Read the model definition and answer for the solid it produces. Units are mm, in the model's axes. Give positions to 0.01 mm unless a question says otherwise; leave off trailing zeros. Write each loop counter-clockwise with the first axis right and the second up, starting at its lowest first coordinate (ties: lowest second). Pieces come first, ordered by that corner, then holes. Notation, with made-up numbers: (32, -18) - (91, -18) arc R30 cw to (91, 5) - close; hole circle Ø2 at (33.5, 50.25). An arc over 180 degrees is marked (long way). Answer as CSV lines item,"result".
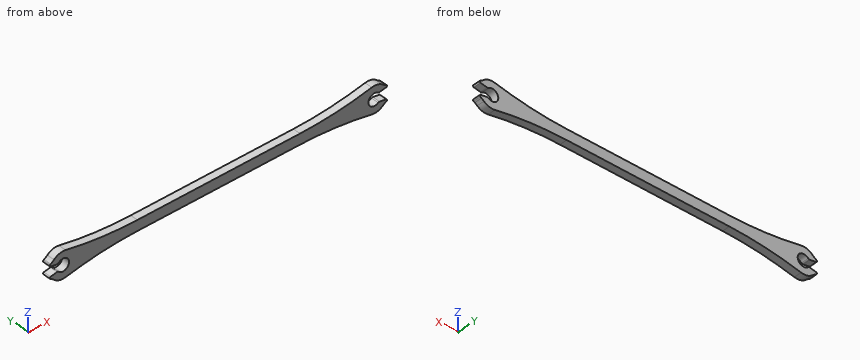
```python
from build123d import *

# Parameters (mm, degrees)
F1_DEPTH = 1.1
F2_R     = 0.3
F3_R     = 100
F4_R     = 0.5
F5_R     = 5


with BuildPart() as f1:
    # F0 (on Front) → F1 (new body, symmetric)
    with BuildSketch(Plane.XZ):
        with BuildLine():
            ThreePointArc((1.224745, -1.25), (-1.75, 0), (1.224745, 1.25))
            Line((1.224745, 1.25), (4.179168, 1.770945))
            Line((4.179168, 1.770945), (2.648788, 2.65451))
            ThreePointArc((2.648788, 2.65451), (-0.698939, 3.684289), (-3.436932, 1.5))
            Line((-3.436932, 1.5), (-86.563068, 1.5))
            ThreePointArc((-86.563068, 1.5), (-89.480722, 3.713873), (-92.893705, 2.385156))
            Line((-92.893705, 2.385156), (-94.390564, 1.520945))
            Line((-94.390564, 1.520945), (-91.436141, 1))
            ThreePointArc((-91.436141, 1), (-88.25, 0), (-91.436141, -1))
            Line((-91.436141, -1), (-94.390564, -1.520945))
            Line((-94.390564, -1.520945), (-92.893705, -2.385156))
            ThreePointArc((-92.893705, -2.385156), (-89.480722, -3.713873), (-86.563068, -1.5))
            Line((-86.563068, -1.5), (-3.436932, -1.5))
            ThreePointArc((-3.436932, -1.5), (-0.698939, -3.684289), (2.648788, -2.65451))
            Line((2.648788, -2.65451), (4.179168, -1.770945))
            Line((4.179168, -1.770945), (1.224745, -1.25))
        make_face()
    extrude(amount=F1_DEPTH, both=True)

    # F2
    f2_edges = [f1.edges().sort_by_distance(p)[0] for p in [
        (4.179168, 0, 1.770945),
        (4.179168, 0, -1.770945),
        (-94.390564, 0, -1.520945),
        (-94.390564, 0, 1.520945),
    ]]
    fillet(f2_edges, radius=F2_R)

    # F3
    f3_edges = [f1.edges().sort_by_distance(p)[0] for p in [
        (-3.436932, 0, 1.5),
        (-3.436932, 0, -1.5),
        (-86.563068, 0, 1.5),
        (-86.563068, 0, -1.5),
    ]]
    fillet(f3_edges, radius=F3_R)

    # F4
    f4_edges = [f1.edges().sort_by_distance(p)[0] for p in [
        (1.224745, 0, 1.25),
        (1.224745, 0, -1.25),
        (-91.436141, 0, 1),
        (-91.436141, 0, -1),
    ]]
    fillet(f4_edges, radius=F4_R)

    # F5
    f5_edges = [f1.edges().sort_by_distance(p)[0] for p in [
        (2.648788, 0, 2.65451),
        (2.648788, 0, -2.65451),
        (-92.893705, 0, -2.385156),
        (-92.893705, 0, 2.385156),
    ]]
    fillet(f5_edges, radius=F5_R)


solid = f1.part
```
(1) Each of these flat-tipped pins is pushed along its axis until it touches: P1, Ø2, axis at x = -90, z = 0, coming from the +Y side; P2, Ø1.1, axis at x = -45, y = 0, coming from the -Z side. Where does it stop, or does it pass through?
Worked out:
P1,"passes through"
P2,"stops at z = -1.5"
(2) Find the intervals of material crossed by L1, parallel to Z at x = 0, y = 0.1; L2, parallel to X at y = -0.4, z = 0; L3, parallel to Z at x = -45.5, y = 0.1, in increasing order.
Worked out:
L1,"z = -3.75 to -1.75, 1.75 to 3.75"
L2,"x = -88.25 to -1.75"
L3,"z = -1.5 to 1.5"
(3) A cutting plane is placed at C-C (x = -62.5). Write down the section's boundary in (y, z).
Worked out:
outline,"(-1.1, -1.5) - (1.1, -1.5) - (1.1, 1.5) - (-1.1, 1.5) - close"
(4) A cutting plane is placed at B-B (z = 0). Write down the section's boundary in (x, y).
Worked out:
outline,"(-88.25, -1.1) - (-1.75, -1.1) - (-1.75, 1.1) - (-88.25, 1.1) - close"
